Geometry check sheet. Reference: drawing and pictorial views, mm from the part's lowest x, y, z. A direction names the side the tool comes from. Coordinates: 2 decimals unless noted, no trailing zeros. Loops run counter-clockwise (first coordinate to the right, second up) from the corner with the lowest first, then second, coordinate; pieces in that order, holes last. Notation, with made-up numbers: (28, 49) -> (59, 49) arc R34 cw to (59, 87) -> close; hole circle Ø5 at (-35.75, -31). An arc over 180 degrees is marked (long way). Answer as a JSON object with one key per item and string values. Group by question number.
Q1. Set-up check for the marked faces 1, 2 and 3: record each of +Z, -Z, +X, -X, +Y, -Y from which the full face is reachable in a straight line by a thin tool's end or side.
Q2. Cross-section at C-C on y = 4.6. Record the boundary of the cut face in (x, z).
Q3. Scan lines: L1, parallel to Z at x = 8, y = 4.9; L2, parallel to Z at x = 8, y = 3.95; L3, parallel to X at y = 0.3, z = 9.5. Record each from-to range of solid material in increasing order.
Q4. Cross-section at B-B on z = 8. Record the boundary of the cut face in (x, y), and give its area (3 significant figures).
Q5. Cross-section at A-A on x = 8. Record the boundary of the cut face in (y, z), and give its area (3 significant figures).
Q6. Cross-section at D-D on x = 13.25. Record the boundary of the cut face in (y, z).
Q7. Release check for a two-part mould opening along X. For the marked faces 4, 5 and 6 record: released by +X, released by -X, zero draft, split by the parting line, or undercut.
Q8. Gauge pin test, flat ends, axial feed: pin 1 Ø3 at (x, y) = (14, 3.5) entering from +Z; pin 2 Ø3 at (x, y) = (11, 1.5) entering from -Z; pin 3 Ø4 at (x, z) = (8, 7) entering from +Y. Record the tip position at first contact, or that the pin passes through.
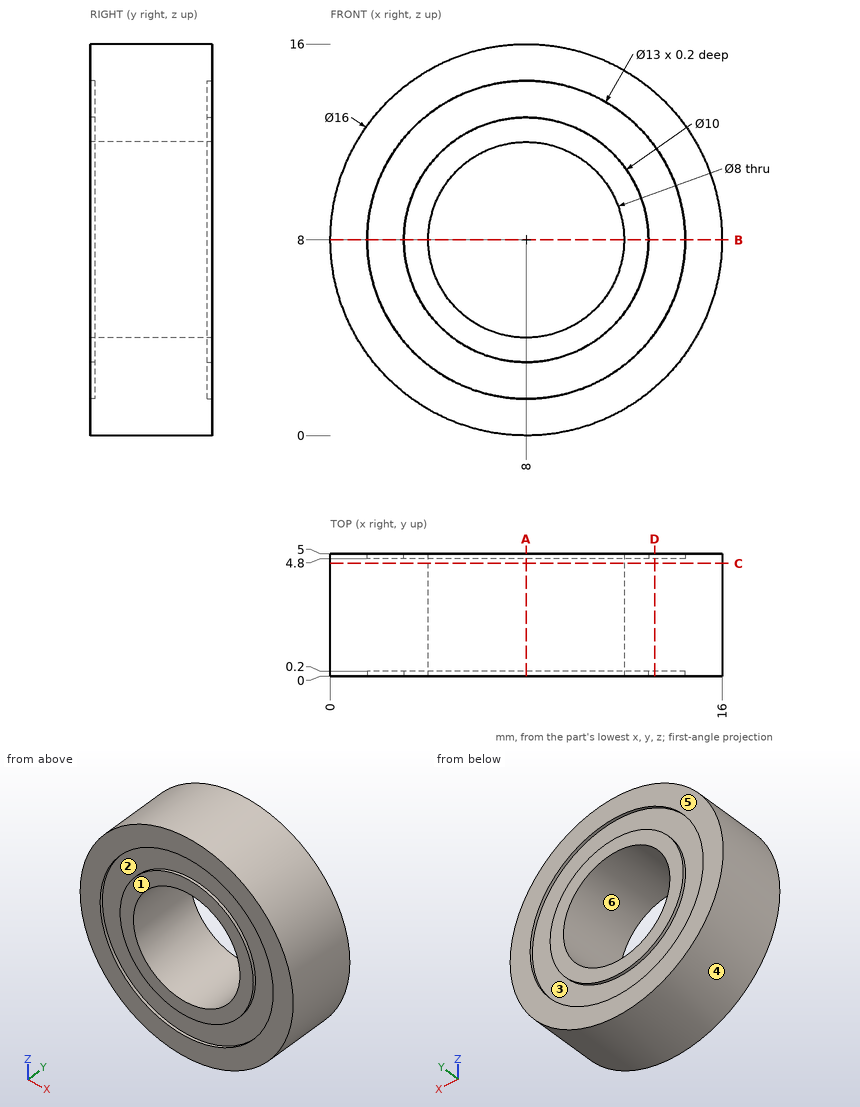
Computed values:
{
 "1": {"face 1": "+Z, -Z, +X, -X, -Y", "face 2": "-Y", "face 3": "+Y"},
 "2": {"outline": "circle Ø16 at (8, 8); hole circle Ø8 at (8, 8)"},
 "3": {"L1": "z = 0 to 1.5, 3 to 4, 12 to 13, 14.5 to 16", "L2": "z = 0 to 4, 12 to 16", "L3": "x = 0.14 to 4.29, 11.71 to 15.86"},
 "4": {"outline": "(0, 0) -> (1.5, 0) -> (1.5, 0.2) -> (3, 0.2) -> (3, 0) -> (4, 0) -> (4, 5) -> (3, 5) -> (3, 4.8) -> (1.5, 4.8) -> (1.5, 5) -> (0, 5) -> close; (12, 0) -> (13, 0) -> (13, 0.2) -> (14.5, 0.2) -> (14.5, 0) -> (16, 0) -> (16, 5) -> (14.5, 5) -> (14.5, 4.8) -> (13, 4.8) -> (13, 5) -> (12, 5) -> close", "area": "38.8 mm²"},
 "5": {"outline": "(0, 0) -> (5, 0) -> (5, 1.5) -> (4.8, 1.5) -> (4.8, 3) -> (5, 3) -> (5, 4) -> (0, 4) -> (0, 3) -> (0.2, 3) -> (0.2, 1.5) -> (0, 1.5) -> close; (0, 12) -> (5, 12) -> (5, 13) -> (4.8, 13) -> (4.8, 14.5) -> (5, 14.5) -> (5, 16) -> (0, 16) -> (0, 14.5) -> (0.2, 14.5) -> (0.2, 13) -> (0, 13) -> close", "area": "38.8 mm²"},
 "6": {"outline": "(0, 1.96) -> (5, 1.96) -> (5, 4.17) -> (4.8, 4.17) -> (4.8, 11.83) -> (5, 11.83) -> (5, 14.04) -> (0, 14.04) -> (0, 11.83) -> (0.2, 11.83) -> (0.2, 4.17) -> (0, 4.17) -> close"},
 "7": {"face 4": "split by the parting line", "face 5": "zero draft", "face 6": "undercut"},
 "8": {"pin 1": "stops at z = 14.61", "pin 2": "stops at z = 0.14", "pin 3": "passes through"}
}
